Part print with two shaded views. Sizes in mm from the minimum x, y, z corner. A direction names the side the tool comes from. Give positions to 0.01 mm unless a question says otherwise; leave off trailing zeros. Write each loop counter-clockwise with the first axis right and the second up, starting at its lowest first coordinate (ties: lowest second). Pieces come first, ordered by that corner, then holes. Notation, with made-up numbers: (9.5, 89.25) -> (18.5, 89.25) arc R12 cw to (18.5, 102.25) -> close; hole circle Ø5 at (5, -33.75). An arc over 180 degrees is marked (long way). Use one line per item in the form item = value. Start each with the question number.
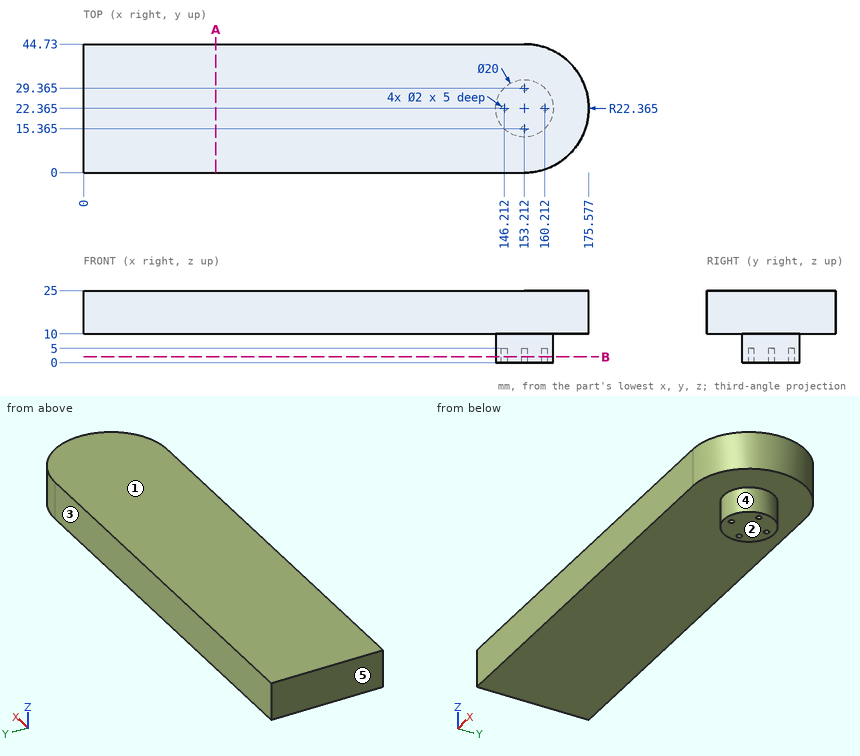
1) Two-plate mould, pull along Z, no slides. Class the marked faces 1, 2 and 3: released by +Z, released by -Z, zero draft, split by the parting line, or undercut.
2) Wall check: line 1 along X through (y, z) = (22.5, 2.5); line 2 along Z through (x, y) = (101, 11); line 3 along X through (y, z) = (28.5, 1) (1 decimal). Give the ranges that are in metal, low to high. Write a range as from..to.
3) 3-axis set-ups, long thin cutter, end or side, ignore diameter. For the marked faces 4 and 5: which of +Z, -Z, +X, -X, +Y, -Y reach the whole face in a straight line?
4) Cut at A-A (x = 46). Give the cut face in (y, z).
5) Cut at B-B (z = 2). Give the cut face in (x, y) (1 decimal).
6) Pin check, flat tips, straight feed: pin 1 (0.6 mm diameter, centred on x = 153, y = 29.5, fed in from -Z); pin 2 (1 mm diameter, centred on x = 57.5, y = 32.5, fed in from -Z); pin 3 (5 mm diameter, centred on y = 29.5, z = 19.5, fed in from +X); pin 4 (4 mm diameter, centred on y = 8, z = 7, fed in from +X). Stop position of each tip, or through.
Final values:
q1.face_1 = released by +Z
q1.face_2 = released by -Z
q1.face_3 = zero draft
q2.line_1 = 143.21..145.22, 147.2..159.22, 161.2..163.21
q2.line_2 = 10..25
q2.line_3 = 145.3..152.7, 153.7..161.1
q3.face_4 = -Z
q3.face_5 = +Z, -Z, -X, +Y, -Y
q4.outline = (0, 10) -> (44.73, 10) -> (44.73, 25) -> (0, 25) -> close
q5.outline = circle Ø20 at (153.2, 22.4); hole circle Ø2 at (146.2, 22.4); hole circle Ø2 at (153.2, 15.4); hole circle Ø2 at (153.2, 29.4); hole circle Ø2 at (160.2, 22.4)
q6.pin_1 = 5
q6.pin_2 = 10
q6.pin_3 = 175.09
q6.pin_4 = through
